The model under review builds one solid part; all positions refer to its coordinate system, in mm. A direction names the side the tool comes from. Give positions to 0.01 mm unless a question says otherwise; leave off trailing zeros. Write each loop counter-clockwise with the first axis right and the second up, starting at its lowest first coordinate (ties: lowest second). Pieces come first, ordered by that corner, then holes. Notation, with made-up numbers: (83.5, -31) - (94.5, -31) arc R15 ccw to (94.5, -8) - close; hole circle Ø7 at (6.5, 19). An arc over 180 degrees is marked (long way). One line per question, with ' | ' between items. Start each with the question number.
```python
from build123d import *

# Parameters (mm, degrees)
SKETCH1_R           = 4
BOSS_EXTRUDE1_DEPTH = 10
FILLET1_R           = 2
SKETCH2_R           = 1.5
CUT_EXTRUDE1_DEPTH  = 65.346717088


with BuildPart() as part:
    # Sketch1 → Boss-Extrude1 (new body)
    with BuildSketch(Plane(origin=(0, 0, 0), x_dir=(1, 0, 0), z_dir=(0, 1, 0))):
        with BuildLine():
            Line((19.5, -49.5), (11, -49.5))
            Line((11, -49.5), (11, 0))
            ThreePointArc((11, 0), (0, 11), (-11, 0))
            Line((-11, 0), (-11, -49.5))
            Line((-11, -49.5), (-19.5, -49.5))
            Line((-19.5, -49.5), (-19.5, -57.5))
            Line((-19.5, -57.5), (19.5, -57.5))
            Line((19.5, -57.5), (19.5, -49.5))
        make_face()
        Polygon((0, -32.265564437), (8.133963179, -46.5), (-8.133963179, -46.5), align=None, mode=Mode.SUBTRACT)
        Polygon((-8, -42.234435563), (-8, -18.265564437), (-1.151751107, -30.25), align=None, mode=Mode.SUBTRACT)
        Polygon((8, -18.265564437), (8, -42.234435563), (1.151751107, -30.25), align=None, mode=Mode.SUBTRACT)
        Polygon((0, -28.234435563), (-8.133963179, -14), (8.133963179, -14), align=None, mode=Mode.SUBTRACT)
        with Locations(Location((0, 0, 0), (0, 0, 270))):
            Circle(SKETCH1_R, mode=Mode.SUBTRACT)
    extrude(amount=BOSS_EXTRUDE1_DEPTH)

    # Fillet1
    fillet1_edges = [part.edges().sort_by_distance(p)[0] for p in [
        (8.133963179, 5, 14),
        (-8.133963179, 5, 14),
        (0, 5, 28.234435563),
        (8, 5, 18.265564437),
        (1.151751107, 5, 30.25),
        (8, 5, 42.234435563),
        (-1.151751107, 5, 30.25),
        (-8, 5, 18.265564437),
        (-8, 5, 42.234435563),
        (8.133963179, 5, 46.5),
        (-8.133963179, 5, 46.5),
        (11, 5, 49.5),
        (19.5, 5, 49.5),
        (19.5, 5, 57.5),
        (-19.5, 5, 57.5),
        (-19.5, 5, 49.5),
        (-11, 5, 49.5),
    ]]
    fillet(fillet1_edges, radius=FILLET1_R)

    # Sketch2 → Cut-Extrude1 (cut, through all)
    with BuildSketch(Plane(origin=(0, 0, 49.5), x_dir=(-1, 0, 0), z_dir=(0, 0, -1))):
        with Locations((-15.25, 5)):
            Circle(SKETCH2_R)
        with Locations((15.25, 5)):
            Circle(SKETCH2_R)
    extrude(amount=-CUT_EXTRUDE1_DEPTH, mode=Mode.SUBTRACT)


solid = part.part
```
Item 1: The part is to be moulded in two halves that separate along X. For faces 1 (the flat face through (-19.5, 5, 53)), 2 (the flat face through (-2.973, 4.93, 33.438)), 3 (the flat face through (0, 10, 30)), say which applies: +X half, -X half, draft (parallel to the pull), parting line (faces both ways), or undercut.
Item 2: Take a section at C-C (z = 8). Give the boundary of the cut face in (x, y), plus the area to 3 significant figures.
Item 3: Take a section at B-B (y = 5). State how many separate pieces and enclosed holes the cut face has, plus the area to 3 significant figures.
Item 4: For probe 1 along X at (y, z) = (1.75, 28.5); probe 2 along Z at (x, y) = (-1, 4.75); probe 3 along X at (y, z) = (5, 30.5), list the stretches that pass through material, from the lowest coordinate up.
Item 5: Clearance check with flat-ended pins moving along their axes: P1, Ø5, axis at x = -15.5, y = 3, coming from the -Z side; P2, Ø6, axis at y = 8, z = -2.5, coming from the +X side; P3, Ø2.5, axis at y = 4.5, z = 32, coming from the -X side; P4, Ø2.5, axis at x = 15.25, y = 5, coming from the -Z side. State where each tip first meets the part, or that it passes through.
Item 6: Take a section at A-A (x = -15.25). Give the boundary of the cut face in (y, z).
Item 7: Machinability: for faces 4 (the flat face through (11, 5, 24)), 5 (the cylindrical face through (0, 5, -11)), 6 (the cylindrical face through (0.029, 5.07, 26.203)), 7 (the flat face through (-11, 5, 23)), which of the approach directions +Z, -Z, +X, -X, +Y, -Y give a long, thin tool a straight path to every point of the face, cutting with its end or side? Answer none if there is none.
Check sheet entries:
1) face 1: -X half | face 2: undercut | face 3: draft
2) outline: (-11, 0) - (11, 0) - (11, 10) - (-11, 10) - close | area: 220 mm^2
3) separate pieces: 3 | enclosed holes: 5 | area: 1,150 mm^2
4) probe 1: x = -11 to -8, -2.15 to 2.15, 8 to 11 | probe 2: z = -10.95 to -3.87, 3.87 to 14, 25.94 to 34.02, 46.5 to 57.5 | probe 3: x = -11 to -8, -1.47 to 1.47, 8 to 11
5) P1: stops at z = 49.5 | P2: stops at x = 11 | P3: stops at x = -11 | P4: passes through
6) outline: (0, 49.5) - (3.5, 49.5) - (3.5, 57.5) - (0, 57.5) - close; (6.5, 49.5) - (10, 49.5) - (10, 57.5) - (6.5, 57.5) - close
7) face 4: -Z, +X, +Y, -Y | face 5: -Z, +Y, -Y | face 6: +Y, -Y | face 7: -Z, -X, +Y, -Y
